Here's how the part is built. I have some questions about the finished solid (model axes, mm). A direction names the side the tool comes from. Coordinates: 2 decimals unless noted, no trailing zeros. Order: outer loops, then holes, each group sorted by start corner. A loop starts at its lowest first (then second) coordinate and runs counter-clockwise, first axis right, second up. Notation, with made-up numbers: (-17, -23.75) - (8, -23.75) arc R28 ccw to (8, 15.25) - close; hole circle Ø5 at (-12, 49.5). An arc over 180 degrees is marked (long way). Answer in a Markdown table with one row per item. Add a question column.
Item 1: I want a section at C-C (x = 32). Please give me the cut outline in (y, z).
Item 2: Will these pins go through, and if not, where does the flat tip stop? pin 1 Ø1.1 at (x, y) = (38, -2) entering from -Z; pin 2 Ø1.5 at (x, y) = (32, -1.5) entering from +Z; pin 3 Ø0.8 at (y, z) = (-1.5, -1.5) entering from -X.
Item 3: I want a section at D-D (z = -2). Please give me the cut outline in (x, y).
Item 4: On a 3-axis mill with a long thin cutter (end or side, diameter ignored), from which of +Z, -Z, +X, -X, +Y, -Y can I reach the whole of each face in a straight line? I mean faces 4 (the flat face through (31, -2.8, 2)), 5 (the flat face through (44, -1, -4.681)), 6 (the flat face through (38, -1, 1.833)). Say none if no direction works.
Item 5: I want a section at B-B (z = -4.25). Please give me the cut outline in (x, y).
Item 6: If I drill on line 1 along X through (y, z) = (-1.45, -3.5); line 2 along X through (y, z) = (-0.9, 0.5); line 3 along Z through (x, y) = (23.5, -2.15), over which ranges is the centre line in solid material (lowest first)? Write a range as from..to.
Item 7: I want a section at A-A (y = -2.25). Please give me the cut outline in (x, z), plus the area to 3 significant figures.
Item 8: Thinking about a two-plate mould opening in X: for faces 1 (the flat face through (31, -0.2, 2)), 2 (the flat face through (47.663, -1, -1)), 3 (the flat face through (40.393, -1, -1)), which applies, +X half, -X half, draft (parallel to the pull), parting line (faces both ways), or undercut?
```python
from build123d import *

# Parameters (mm, degrees)
BOSS_EXTRUDE1_START = -0.2
BOSS_EXTRUDE1_DEPTH = 2.6


with BuildPart() as part:
    # Sketch3 → Boss-Extrude1 (new body)
    with BuildSketch(Plane(origin=(0, 0, 0), x_dir=(1, 0, 0), z_dir=(0, 1, 0)).offset(BOSS_EXTRUDE1_START)):
        with BuildLine():
            Line((24.837294245, -10.53319149), (37.637975917, -10.56578536))
            ThreePointArc((37.637975917, -10.56578536), (44.725498152, -7.645882227), (47.663438439, -0.565817777))
            Line((47.663438439, -0.565817777), (47.663438439, 2.68092068))
            ThreePointArc((47.663438439, 2.68092068), (47.077652002, 4.095134243), (45.663438439, 4.68092068))
            Line((45.663438439, 4.68092068), (42.393317115, 4.68092068))
            ThreePointArc((42.393317115, 4.68092068), (40.979103553, 4.095134243), (40.393317115, 2.68092068))
            Line((40.393317115, 2.68092068), (40.393317115, 0.166619972))
            ThreePointArc((40.393317115, 0.166619972), (39.807530678, -1.24759359), (38.393317115, -1.833380028))
            Line((38.393317115, -1.833380028), (37.396232536, -1.833380028))
            ThreePointArc((37.396232536, -1.833380028), (35.991450888, -1.256963015), (35.396409281, 0.14003145))
            ThreePointArc((35.396409281, 0.14003145), (17.376079319, 7.407980257), (24.837294245, -10.53319149))
        make_face()
    extrude(amount=-BOSS_EXTRUDE1_DEPTH)


solid = part.part
```
Values follow:
| question | item | result |
|---|---|---|
| 1 | outline | (-2.8, -7.75) - (-0.2, -7.75) - (-0.2, 10.55) - (-2.8, 10.55) - close |
| 2 | pin 1 | stops at z = 1.83 |
| 2 | pin 2 | stops at z = 10.55 |
| 2 | pin 3 | stops at x = 14.39 |
| 3 | outline | (14.52, -2.8) - (35.21, -2.8) - (35.21, -0.2) - (14.52, -0.2) - close; (40.39, -2.8) - (47.66, -2.8) - (47.66, -0.2) - (40.39, -0.2) - close |
| 4 | face 4 | +Z, -Z, +X, -X, -Y |
| 4 | face 5 | -Z, +X, +Y, -Y |
| 4 | face 6 | -Z, +Y, -Y |
| 5 | outline | (15.23, -2.8) - (34.5, -2.8) - (34.5, -0.2) - (15.23, -0.2) - close; (41.15, -2.8) - (46.9, -2.8) - (46.9, -0.2) - (41.15, -0.2) - close |
| 6 | line 1 | x = 14.93..34.8, 40.57..47.49 |
| 6 | line 2 | x = 14.34..35.51, 40.28..47.66 |
| 6 | line 3 | z = -10.44..10.44 |
| 7 | outline | (24.84, 10.53) arc R10.53 ccw (long way) to (35.4, -0.14) arc R2 cw to (37.4, 1.83) - (38.39, 1.83) arc R2 cw to (40.39, -0.17) - (40.39, -2.68) arc R2 ccw to (42.39, -4.68) - (45.66, -4.68) arc R2 ccw to (47.66, -2.68) - (47.66, 0.57) arc R10 ccw to (37.64, 10.57) - close |
| 7 | area | 506 mm^2 |
| 8 | face 1 | draft |
| 8 | face 2 | +X half |
| 8 | face 3 | undercut |
